Read the model definition and answer for the solid it produces. Units are mm, in the model's axes. A direction names the side the tool comes from. Coordinates: 2 decimals unless noted, no trailing zeros. Order: outer loops, then holes, each group sorted by start corner. A loop starts at its lowest first (then second) coordinate and runs counter-clockwise, first axis right, second up. Notation, with made-up numbers: (16.5, 83) -> (54.5, 83) arc R10 ccw to (54.5, 99) -> close; hole circle Ø6 at (-36, 83.5). An arc over 180 degrees is marked (long way). Return JSON: item names as keys, results as strings. Group by question number.
```python
from build123d import *

# Parameters (mm, degrees)
BOSS_EXTRUDE1_DEPTH = 6.5
CUT_EXTRUDE3_DEPTH  = 68.659163459
SKETCH4_W           = 4
SKETCH4_H           = 55
SKETCH4_W_2         = 1.7
SKETCH4_H_2         = 62
CUT_EXTRUDE4_DEPTH  = 4.5
SKETCH5_R           = 1.15
BOSS_EXTRUDE2_DEPTH = 2
FILLET1_R           = 1.5
CUT_EXTRUDE5_REACH  = 36.8
SKETCH7_W           = 5.32
SKETCH7_H           = 0.3
SKETCH6_R           = 1.4
CUT_EXTRUDE6_DEPTH  = 2.8
FILLET2_R           = 1.5
FILLET3_R           = 1.5
CUT_EXTRUDE7_REACH  = 37.922
CUT_EXTRUDE8_START  = -2.451564
SKETCH10_RX         = 1.15
SKETCH10_RY         = 0.8
CUT_EXTRUDE8_DEPTH  = 2.451564


with BuildPart() as part:
    # Sketch1 → Boss-Extrude1 (new body)
    with BuildSketch(Plane(origin=(0, 0, 0), x_dir=(1, 0, 0), z_dir=(0, 1, 0))):
        Polygon((1.5, -31), (6.82, -31), (6.82, 31), (1.5, 31), (1.5, 33.5), (-5.5, 33.5), (-5.5, 31), (-1.2, 31), (-1.2, -31), (-5.5, -31), (-5.5, -33.5), (1.5, -33.5), align=None)
    extrude(amount=-BOSS_EXTRUDE1_DEPTH)

    # Sketch3 → Cut-Extrude3 (cut, through all)
    with BuildSketch(Plane.XY.offset(33.5)):
        with BuildLine():
            Line((-5.5, 0), (-5.5, -3.25))
            ThreePointArc((-5.5, -3.25), (-4.548097039, -0.951902961), (-2.25, 0))
            Line((-2.25, 0), (-5.5, 0))
        make_face()
        with BuildLine():
            Line((-5.5, -6.5), (-2.25, -6.5))
            ThreePointArc((-2.25, -6.5), (-4.548097039, -5.548097039), (-5.5, -3.25))
            Line((-5.5, -3.25), (-5.5, -6.5))
        make_face()
    extrude(amount=-CUT_EXTRUDE3_DEPTH, mode=Mode.SUBTRACT)

    # Sketch4 → Cut-Extrude4 (cut)
    with BuildSketch(Plane.XZ.offset(6.5)):
        with Locations((4.82, 0)):
            Rectangle(SKETCH4_W, SKETCH4_H)
        with Locations((-0.35, 0)):
            Rectangle(SKETCH4_W_2, SKETCH4_H_2)
    extrude(amount=-CUT_EXTRUDE4_DEPTH, mode=Mode.SUBTRACT)

    # Sketch5 → Boss-Extrude2 (add)
    with BuildSketch(Plane.XY.offset(-31)):
        with Locations((-3.25, -3.25)):
            Circle(SKETCH5_R)
    boss_extrude2 = extrude(amount=BOSS_EXTRUDE2_DEPTH)

    # Fillet1
    fillet1_edges = [part.edges().sort_by_distance(p)[0] for p in [
        (-1.2, -2, 0),
    ]]
    fillet(fillet1_edges, radius=FILLET1_R)

    # Sketch7 → Cut-Extrude5 (cut, up to next)
    with BuildSketch(Plane(origin=(0, 0, 0), x_dir=(1, 0, 0), z_dir=(0, 1, 0)), mode=Mode.PRIVATE) as cut_extrude5_sk1:
        with Locations((4.16, 30.85)):
            Rectangle(SKETCH7_W, SKETCH7_H)
    cut_extrude5_tool1 = extrude(cut_extrude5_sk1.sketch, amount=-CUT_EXTRUDE5_REACH, mode=Mode.PRIVATE) & part.part
    cut_extrude5 = cut_extrude5_tool1.solids().sort_by_distance((4.16, 0, -30.85))[0]
    add(cut_extrude5, mode=Mode.SUBTRACT)

    # Sketch6 → Cut-Extrude6 (cut)
    with BuildSketch(Plane(origin=(0, 0, -31), x_dir=(-1, 0, 0), z_dir=(0, 0, -1))):
        with Locations((-5.07, -3.25)):
            Circle(SKETCH6_R)
    cut_extrude6 = extrude(amount=-CUT_EXTRUDE6_DEPTH, mode=Mode.SUBTRACT)

    # Mirror2: Boss-Extrude2, Cut-Extrude5, Cut-Extrude6 across plane
    add(boss_extrude2.mirror(Plane.XY))
    add(cut_extrude5.mirror(Plane.XY), mode=Mode.SUBTRACT)
    add(cut_extrude6.mirror(Plane.XY), mode=Mode.SUBTRACT)

    # Fillet2
    fillet2_edges = [part.edges().sort_by_distance(p)[0] for p in [
        (6.82, -2, 0),
    ]]
    fillet(fillet2_edges, radius=FILLET2_R)

    # Fillet3
    fillet3_edges = [part.edges().sort_by_distance(p)[0] for p in [
        (6.82, -6.5, 29.1),
        (6.82, -6.5, -29.1),
    ]]
    fillet(fillet3_edges, radius=FILLET3_R)

    # Sketch9 → Cut-Extrude7 (cut, up to next)
    with BuildSketch(Plane.ZY.offset(4.4), mode=Mode.PRIVATE) as cut_extrude7_sk1:
        Polygon((-29, -3.95), (-29.9, -2.1), (-29, -2.1), align=None)
    cut_extrude7_tool1 = extrude(cut_extrude7_sk1.sketch, amount=-CUT_EXTRUDE7_REACH, mode=Mode.PRIVATE) & part.part
    cut_extrude7 = cut_extrude7_tool1.solids().sort_by_distance((-4.4, -2.716667, -29.3))[0]
    add(cut_extrude7, mode=Mode.SUBTRACT)

    # Sketch10 → Cut-Extrude8 (cut)
    with BuildSketch(Plane.XZ.offset(6.5).offset(CUT_EXTRUDE8_START)):
        with Locations(Location((5.07, -30.7), (0, 0, 180))):
            Ellipse(SKETCH10_RX, SKETCH10_RY)
    cut_extrude8 = extrude(amount=CUT_EXTRUDE8_DEPTH, mode=Mode.SUBTRACT)

    # Mirror3: Cut-Extrude7, Cut-Extrude8 across plane
    add(cut_extrude7.mirror(Plane.XY), mode=Mode.SUBTRACT)
    add(cut_extrude8.mirror(Plane.XY), mode=Mode.SUBTRACT)


solid = part.part
```
1. Find section A-A on z = 14.5. Determine the outline of the cut face in (x, y), and give its area (3 significant figures).
2. Which of the six approach directions +Z, -Z, +X, -X, +Y, -Y give full straight-line access (tool end or side, diameter ignored) to faces 1 (the face through (-3.266, -3.038, 29.444)), 2 (the face through (-3.499, -4.373, 30.236)), 3 (the face through (1.5, -3, -32)), 4 (the face through (2.82, -4, 0))?
3. Given pin 1 (1 mm diameter, centred on y = -5.5, z = -13, fed in from -X); pin 2 (0.8 mm diameter, centred on x = 5, y = -3, fed in from +Z); pin 3 (1.5 mm diameter, centred on x = 5, z = 3.5, fed in from -Y), each flat-ended and moving along its own axis, determine where each tip first touches the part or whether it passes through.
4. For a pull along X with two mould halves and no side action, classify faces 5 (the face through (-2, -3, -33.5)), 6 (the face through (-0.77, -1.55, 0.43)), 7 (the face through (-1.9, -3.2, -31)), 8 (the face through (6.39, -6.05, -29.12)) as released by +X, released by -X, zero draft, split by the parting line, or undercut.
5. Straight lines are drawn through the part: L1, parallel to X at y = -3.25, z = 29.7; L2, parallel to Z at x = -2, y = -5; L3, parallel to Y at x = 5.07, z = -28.8. For each, find the intervals that lie inside material, in ascending order.
6. Find section B-B on x = -3.25. Determine the outline of the cut face in (y, z).
Result:
{
 "1": {"outline": "(-1.2, -0.5) arc R1.5 ccw to (0.3, -2) -> (0.5, -2) -> (0.5, -6.5) -> (2.82, -6.5) -> (2.82, -2) -> (5.32, -2) arc R1.5 ccw to (6.82, -0.5) -> (6.82, 0) -> (-1.2, 0) -> close", "area": "25.5 mm^2"},
 "2": {"face 1": "-X, +Y", "face 2": "none", "face 3": "-Z, +X, +Y, -Y", "face 4": "+X, -Y"},
 "3": {"pin 1": "x = 0.5", "pin 2": "z = 28.2", "pin 3": "y = -2"},
 "4": {"face 5": "zero draft", "face 6": "released by -X", "face 7": "undercut", "face 8": "released by +X"},
 "5": {"L1": "-4.4 to -2.1, 0.5 to 3.67, 6.47 to 6.82", "L2": "-33.5 to -31, 31 to 33.5", "L3": "-6.5 to -4.65, -1.85 to 0"},
 "6": {"outline": "(-6.34, -33.5) -> (-0.16, -33.5) -> (-0.16, -31) -> (-2.1, -31) -> (-2.1, -29.9) -> (-3.95, -29) -> (-4.4, -29) -> (-4.4, -31) -> (-6.34, -31) -> close; (-6.34, 31) -> (-4.4, 31) -> (-4.4, 29) -> (-3.95, 29) -> (-2.1, 29.9) -> (-2.1, 31) -> (-0.16, 31) -> (-0.16, 33.5) -> (-6.34, 33.5) -> close"}
}
